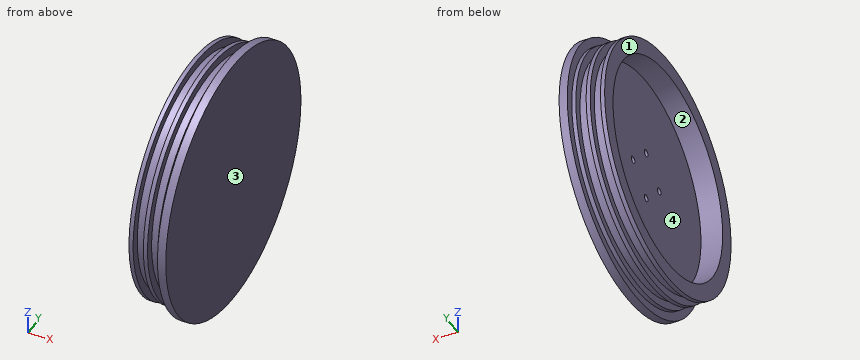
```python
from build123d import *

# Parameters (mm, degrees)
F_6_32_TAPPED_HOLE1_D     = 2.7051
F_6_32_TAPPED_HOLE1_DEPTH = 4.318
F_6_32_TAPPED_HOLE1_TIP   = 0.81269403


with BuildPart() as part:
    # Sketch1 → Revolve1 (revolve)
    with BuildSketch(Plane.XY):
        Polygon((4.318, 50.673), (4.318, 47.371), (2.7305, 47.371), (2.7305, 44.2722), (-1.2065, 44.2722), (-1.2065, 47.371), (-2.794, 47.371), (-2.794, 44.2722), (-6.731, 44.2722), (-6.731, 47.371), (-8.3185, 47.371), (-8.3185, 41.0972), (0, 41.0972), (0, 0), (7.493, 0), (7.493, 50.673), align=None)
    revolve(axis=Axis((0, 0, 0), (1, 0, 0)))

    # #6-32 Tapped Hole1
    with Locations(Plane.ZY):
        with Locations((0, 9.779), (0, -9.779), (-9.779, 0), (9.779, 0)):
            Hole(F_6_32_TAPPED_HOLE1_D / 2, depth=F_6_32_TAPPED_HOLE1_DEPTH)
            with Locations((0, 0, -(F_6_32_TAPPED_HOLE1_DEPTH + F_6_32_TAPPED_HOLE1_TIP / 2))):  # 118° drill point
                Cone(0, F_6_32_TAPPED_HOLE1_D / 2, F_6_32_TAPPED_HOLE1_TIP, mode=Mode.SUBTRACT)


solid = part.part
```
Model file for the job. Use its own axes, mm. Face numbers are marked on the shaded views. A direction names the side the tool comes from. Coordinates: 2 decimals unless noted, no trailing zeros. Loops run counter-clockwise (first coordinate to the right, second up) from the corner with the lowest first, then second, coordinate; pieces in that order, holes last. Notation, with made-up numbers: (-1, -11) - (13, -11) arc R20 ccw to (13, 18) - close; hole circle Ø7 at (43.5, -37). An arc over 180 degrees is marked (long way). Write item = value, one per line. Start each with the question number.
Item 1: Saw through at D-D, the plane x = 1.5. List the corners of the cut face in (y, z).
Item 2: Wall check: probe 1 along Z at (x, y) = (2.05, 0); probe 2 along Y at (x, z) = (-1.75, 0.5); probe 3 along X at (y, z) = (-27, -17). Give the ranges that are in metal, low to high. Write a range as [from, to].
Item 3: Saw through at B-B, the plane y = 19. List the corners of the cut face in (x, z), then the cut area to 3 significant figures.
Item 4: 3-axis set-ups, long thin cutter, end or side, ignore diameter. For the marked faces 1 and 2: which of +Z, -Z, +X, -X, +Y, -Y reach the whole face in a straight line?
Item 5: Saw through at A-A, the plane x = -5. List the corners of the cut face in (y, z), then the cut area to 3 significant figures.
Item 6: Pull direction Y, two halves, no side cores. Call the marked faces 3 and 4: +Y half, -Y half, draft (parallel to the pull), parting line (faces both ways), or undercut.
Item 7: Saw through at C-C, the plane z = -13. List the corners of the cut face in (x, y).
Item 8: Drop flat-ended pins along their axis: pin 1 Ø3 at (x, z) = (3, 12) entering from +Y; pin 2 Ø2 at (y, z) = (11.5, 19) entering from -X; pin 3 Ø1.6 at (y, z) = (0, 9.779) entering from -X. Give the stop position or say it passes through.
Answers:
q1.outline = circle Ø88.54 at (0, 0); hole circle Ø2.71 at (-9.78, 0); hole circle Ø2.71 at (0, -9.78); hole circle Ø2.71 at (0, 9.78); hole circle Ø2.71 at (9.78, 0)
q2.probe_1 = [-44.27, -11.13], [-8.43, 8.43], [11.13, 44.27]
q2.probe_2 = [-47.37, -41.09], [41.09, 47.37]
q2.probe_3 = [0, 7.49]
q3.outline = (-8.32, -43.39) - (-6.73, -43.39) - (-6.73, -39.99) - (-2.79, -39.99) - (-2.79, -43.39) - (-1.21, -43.39) - (-1.21, -39.99) - (2.73, -39.99) - (2.73, -43.39) - (4.32, -43.39) - (4.32, -46.98) - (7.49, -46.98) - (7.49, 46.98) - (4.32, 46.98) - (4.32, 43.39) - (2.73, 43.39) - (2.73, 39.99) - (-1.21, 39.99) - (-1.21, 43.39) - (-2.79, 43.39) - (-2.79, 39.99) - (-6.73, 39.99) - (-6.73, 43.39) - (-8.32, 43.39) - (-8.32, 36.44) - (0, 36.44) - (0, -36.44) - (-8.32, -36.44) - close
q3.area = 735 mm2
q4.face_1 = +Z, -Z, -X, +Y, -Y
q4.face_2 = -X
q5.outline = circle Ø88.54 at (0, 0); hole circle Ø82.19 at (0, 0)
q5.area = 852 mm2
q6.face_3 = draft
q6.face_4 = undercut
q7.outline = (-8.32, -45.55) - (-6.73, -45.55) - (-6.73, -42.32) - (-2.79, -42.32) - (-2.79, -45.55) - (-1.21, -45.55) - (-1.21, -42.32) - (2.73, -42.32) - (2.73, -45.55) - (4.32, -45.55) - (4.32, -48.98) - (7.49, -48.98) - (7.49, 48.98) - (4.32, 48.98) - (4.32, 45.55) - (2.73, 45.55) - (2.73, 42.32) - (-1.21, 42.32) - (-1.21, 45.55) - (-2.79, 45.55) - (-2.79, 42.32) - (-6.73, 42.32) - (-6.73, 45.55) - (-8.32, 45.55) - (-8.32, 38.99) - (0, 38.99) - (0, -38.99) - (-8.32, -38.99) - close
q8.pin_1 = 49.4
q8.pin_2 = 0
q8.pin_3 = 4.65
